Model file for the job. Use its own axes, mm. A direction names the side the tool comes from. Round coordinates to 2 decimals unless told otherwise and drop trailing zeros. Loops run counter-clockwise (first coordinate to the right, second up) from the corner with the lowest first, then second, coordinate; pieces in that order, holes last. Notation, with made-up numbers: M -17,27 L 19,27 A6 ccw 19,35 Z; hole C -26,10 d5. An arc over 180 degrees is marked long. Use a Markdown table: item, result. Add a question column.
Item 1: Wall check: L1, parallel to Z at x = -47.6, y = -74.4; L2, parallel to Z at x = -7.5, y = -79.5; L3, parallel to Y at x = -18, z = 3. Give the ranges that are in metal, low to high. Write a range as from..to.
Item 2: Pin check, flat tips, straight feed: P1, Ø2, axis at x = 31.5, y = -79, coming from the -Z side; P2, Ø1.5, axis at y = -77, z = 3.5, coming from the -X side; P3, Ø3.5, axis at x = 0, y = -78.5, coming from the -Z side. Stop position of each tip, or through.
Item 3: Saw through at A-A on y = -73.75. Write the cut outline in (x, z).
Item 4: Saw through at C-C on z = -4. Write the cut outline in (x, y), then the cut area to 3 significant figures.
Item 5: Two-plate mould, pull along Z, no slides. Class faces 1 (the flat face through (-1, -71.8, -6)), 2 (the flat face through (0, -77, 5.369)), 3 (the flat face through (-5.425, -79.35, -3.074)): +Z half, -Z half, draft (parallel to the pull), parting line (faces both ways), or undercut.
Item 6: Saw through at B-B on x = -47.6. Write the cut outline in (y, z).
Item 7: Saw through at D-D on x = 21.5. Write the cut outline in (y, z).
Item 8: Tool access for faces 4 (the flat face through (-5.375, -79.35, 3.161)), 5 (the flat face through (5.375, -79.35, -3.161)), 6 (the flat face through (4.63, -77.32, -2.72)), 7 (the flat face through (5.425, -79.35, 3.074)): list every direction of +Z, -Z, +X, -X, +Y, -Y with a clear straight run to the whole face (end or side of a thin tool).
```python
from build123d import *

# Parameters (mm, degrees)
SKETCH003_R             = 1.6
PAD003_DEPTH            = 4
SKETCH033_W             = 89.681574
SKETCH033_H             = 0.835685
PAD026_DEPTH            = 6
PAD033_DEPTH            = 7.2
BODY002_PLACEMENT_ANGLE = 180


with BuildPart() as part:
    # Sketch003 → Pad003 (new body)
    with BuildSketch(Plane.XZ):
        with BuildLine():
            Line((-49.09338, 7.071068), (49.09338, 7.071068))
            ThreePointArc((49.09338, -7.071068), (49.6, 0), (49.09338, 7.071068))
            Line((-49.09338, -7.071068), (49.09338, -7.071068))
            ThreePointArc((-49.09338, 7.071068), (-49.6, 0), (-49.09338, -7.071068))
        make_face()
        with Locations((47.6, 0)):
            Circle(SKETCH003_R, mode=Mode.SUBTRACT)
        with Locations((-47.6, 0)):
            Circle(SKETCH003_R, mode=Mode.SUBTRACT)
        Polygon((6.2, 0), (3.1, 5.369358), (-3.1, 5.369358), (-6.2, 0), (-3.1, -5.369358), (3.1, -5.369358), align=None, mode=Mode.SUBTRACT)
    extrude(amount=PAD003_DEPTH)

    # Sketch033 → Pad026 (join)
    with BuildSketch(Plane(origin=(0, 0, 0), x_dir=(1, 0, 0), z_dir=(0, 1, 0))):
        with Locations((0, -6.653225)):
            Rectangle(SKETCH033_W, SKETCH033_H)
    extrude(amount=PAD026_DEPTH)

    # Sketch028 (on Face4 of Pad026) → Pad033 (join)
    with BuildSketch(Plane(origin=(0, 0, 0), x_dir=(1, 0, 0), z_dir=(0, 1, 0))):
        Polygon((3.6, 6.235383), (-3.6, 6.235383), (-7.2, 0), (-3.6, -6.235383), (3.6, -6.235383), (7.2, 0), align=None)
        Polygon((3.1, 5.369358), (-3.1, 5.369358), (-6.2, 0), (-3.1, -5.369358), (3.1, -5.369358), (6.2, 0), align=None, mode=Mode.SUBTRACT)
    extrude(amount=PAD033_DEPTH)


with BuildPart() as part_1:
    # Body002 placement: moved
    add(part.part.moved(Location((0, -75.8, 0))).rotate(Axis((0, -75.8, 0), (0, 0, 1)), BODY002_PLACEMENT_ANGLE))


solid = part_1.part
```
Entries:
| question | item | result |
|---|---|---|
| 1 | L1 | -7.07..-1.6, 1.6..7.07 |
| 1 | L2 | 6.24..7.07 |
| 1 | L3 | -75.8..-71.8 |
| 2 | P1 | z = 6.24 |
| 2 | P2 | x = -5.61 |
| 2 | P3 | z = -6.24 |
| 3 | outline | M -49.09,-7.07 L 49.09,-7.07 A49.6 ccw 49.09,7.07 L -49.09,7.07 A49.6 ccw Z; hole C -47.6,0 d3.2; hole M -6.2,0 L -3.1,-5.37 L 3.1,-5.37 L 6.2,0 L 3.1,5.37 L -3.1,5.37 Z; hole C 47.6,0 d3.2 |
| 4 | outline | M -49.44,-75.8 L -4.89,-75.8 L -4.89,-83 L -3.89,-83 L -3.89,-71.8 L -49.44,-71.8 Z; M 3.89,-83 L 4.89,-83 L 4.89,-75.8 L 49.44,-75.8 L 49.44,-71.8 L 3.89,-71.8 Z |
| 4 | area | 379 mm2 |
| 5 | face 1 | draft |
| 5 | face 2 | undercut |
| 5 | face 3 | -Z half |
| 6 | outline | M -75.8,-7.07 L -71.8,-7.07 L -71.8,-1.6 L -75.8,-1.6 Z; M -75.8,1.6 L -71.8,1.6 L -71.8,7.07 L -75.8,7.07 Z |
| 7 | outline | M -81.8,6.24 L -75.8,6.24 L -75.8,-7.07 L -71.8,-7.07 L -71.8,7.07 L -81.8,7.07 Z |
| 8 | face 4 | -X, -Y |
| 8 | face 5 | -Z, +X, -Y |
| 8 | face 6 | +Y, -Y |
| 8 | face 7 | +X, -Y |
